```python
from build123d import *

# Parameters (mm, degrees)
EXTRUDE1_DEPTH                            = 139.7
F_29_32_0_90625_DIAMETER_HOLE1_AT_2_COUNT = 2
F_29_32_0_90625_DIAMETER_HOLE1_AT_2_PITCH = 93.472


with BuildPart() as part:
    # Sketch1 → Extrude1 (new body)
    with BuildSketch(Plane.XY):
        with BuildLine():
            Line((-25.4, 0), (-25.4, 26.67))
            Line((-25.4, 26.67), (25.4, 26.67))
            Line((25.4, 26.67), (25.4, 0))
            ThreePointArc((25.4, 0), (0, -25.4), (-25.4, 0))
        make_face()
    extrude(amount=EXTRUDE1_DEPTH)

    # Sketch2 → 29/32 (0.90625) Diameter Hole1 (revolve, cut)
    with BuildSketch(Plane(origin=(0, 26.67, 23.114), x_dir=(0, 0, 1), z_dir=(1, 0, 0))):
        Polygon((0, 0), (0, 52.07), (12.2682, 52.07), (11.509375, 51.311175), (11.509375, 0.758825), (12.2682, 0), align=None)
    f_29_32_0_90625_diameter_hole1 = revolve(axis=Axis((0, 33.02, 23.114), (0, -1, 0)), mode=Mode.SUBTRACT)

    # 29/32 (0.90625) Diameter Hole1 at 2: 29/32 (0.90625) Diameter Hole1 ×2
    with Locations(*[(0, 0, i * F_29_32_0_90625_DIAMETER_HOLE1_AT_2_PITCH) for i in range(1, F_29_32_0_90625_DIAMETER_HOLE1_AT_2_COUNT)]):
        add(f_29_32_0_90625_diameter_hole1, mode=Mode.SUBTRACT)


solid = part.part
```
Read the model definition and answer for the solid it produces. Units are mm, in the model's axes. A direction names the side the tool comes from. Give positions to 0.01 mm unless a question says otherwise; leave off trailing zeros. Loops run counter-clockwise (first coordinate to the right, second up) from the corner with the lowest first, then second, coordinate; pieces in that order, holes last.
Item 1: The part is cut by section B-B (z = 103). Write down the section's boundary in (x, y).
Item 2: The part is cut by section A-A (y = 9.5). Write down the section's boundary in (x, z).
Item 3: For faces 1 (the conical face through (-0.09, -24.76, 104.96)), 2 (the cylindrical face through (-3.457, 0.989, 127.564)), determine the directions among +Z, -Z, +X, -X, +Y, -Y from which every point of the face is accessible in a straight line to the end or side of a thin tool.
Item 4: Each of these flat-tipped pins is pushed along its axis until it touches: pin 1 Ø8 at (y, z) = (-16.5, 52.5) entering from +X; pin 2 Ø5 at (x, z) = (-8.5, 16.5) entering from -Y; pin 3 Ø8 at (x, z) = (-2.5, 18) entering from +Y; pin 4 Ø3 at (x, y) = (19, -3) entering from -Z. Where does it stop, or does it pass through?
Item 5: The mould has two halves that part along X. Classify faces 3 (the conical face through (0.092, -24.762, 128.216)), 4 (the flat face through (0, 26.67, 69)), 5 (the flat face through (-25.4, 13, 69)): released by +X, released by -X, zero draft, split by the parting line, or undercut.
Item 6: The part is cut by section D-D (x = 15.5). Write down the section's boundary in (y, z).
Item 7: The part is cut by section C-C (x = -10). Give the number of separate pieces and of enclosed holes in the cut face, and give its area (3 significant figures).
Item 8: Find the intervals of material crossed by line 1 along Z through (x, y) = (0, 14.5); line 2 along Z through (x, y) = (-8, -21.5); line 3 along X through (y, z) = (20, 124.5), in increasing order.
Taken from the geometry:
1. outline: (-25.4, 0) arc R25.4 ccw to (25.4, 0) - (25.4, 26.67) - (-25.4, 26.67) - close
2. outline: (-25.4, 0) - (25.4, 0) - (25.4, 139.7) - (-25.4, 139.7) - close; hole circle Ø23.02 at (0, 23.11); hole circle Ø23.02 at (0, 116.59)
3. face 1: -Y
3. face 2: +Y, -Y
4. pin 1: stops at x = 22.11
4. pin 2: stops at y = -24.31
4. pin 3: passes through
4. pin 4: stops at z = 0
5. face 3: undercut
5. face 4: zero draft
5. face 5: released by -X
6. outline: (-20.12, 0) - (26.67, 0) - (26.67, 139.7) - (-20.12, 139.7) - close
7. separate pieces: 3
7. enclosed holes: 0
7. area: 5,850 mm2
8. line 1: z = 0 to 11.6, 34.62 to 105.08, 128.1 to 139.7
8. line 2: z = 0 to 14.84, 31.39 to 108.31, 124.86 to 139.7
8. line 3: x = -25.4 to -8.36, 8.36 to 25.4
